Check sheet for the drawn part. Datum: minimum x, y, z corner. Units: mm. Give positions to 0.01 mm unless a question says otherwise; leave off trailing zeros. Order: outer loops, then holes, each group sorted by start corner. A loop starts at its lowest first (then second) coordinate and runs counter-clockwise, first axis right, second up.
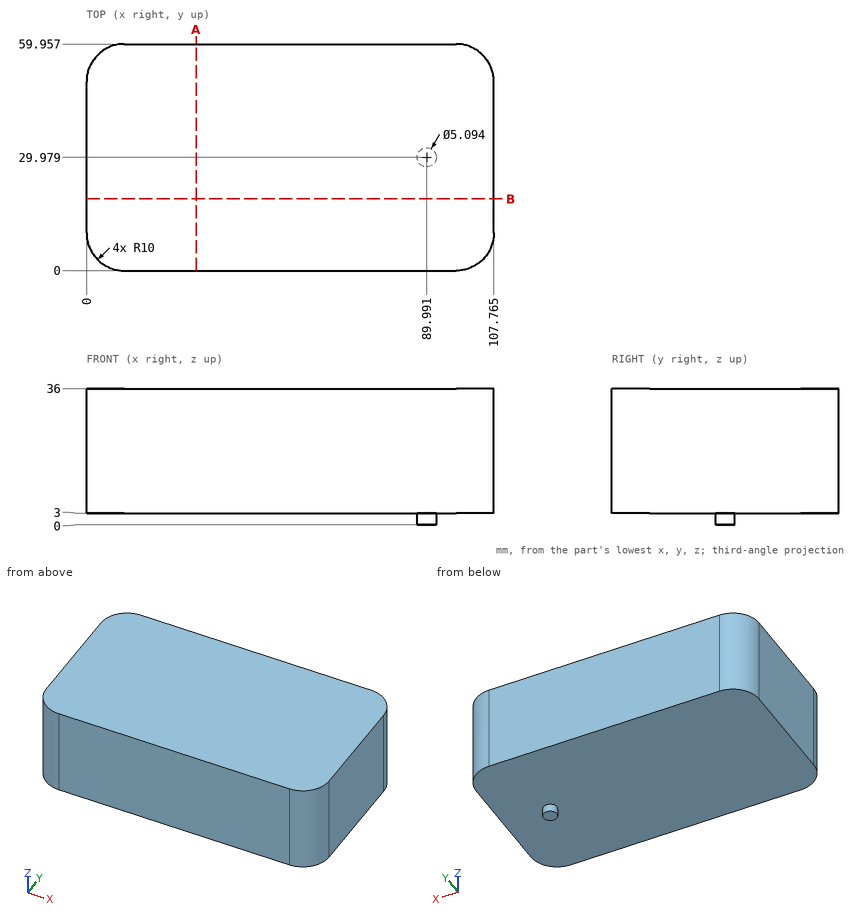
Item 1: Scan lines: L1, parallel to Z at x = 47.5, y = 47.5; L2, parallel to Y at x = 90, z = 2.5 (1 decimal); L3, parallel to Y at x = 8, z = 14 (1 decimal). Record each from-to range of solid material in increasing order.
Reported:
L1: z = 3 to 36
L2: y = 27.4 to 32.5
L3: y = 0.2 to 59.8
Item 2: Sectioned sample at A-A (x = 29). Enter the section's corners in (y, z).
Reported:
outline: (0, 3) - (59.96, 3) - (59.96, 36) - (0, 36) - close
Item 3: Sectioned sample at B-B (y = 19). Enter the section's corners in (x, z) (1 decimal).
Reported:
outline: (0, 3) - (107.8, 3) - (107.8, 36) - (0, 36) - close
Item 4: Gauge pin test, flat end, axial feed: pin 1 (18 mm diameter, centred on x = 76.5, y = 16, fed in from -Z). Record the tip position at first contact, or that the pin passes through.
Reported:
pin 1: stops at z = 3
